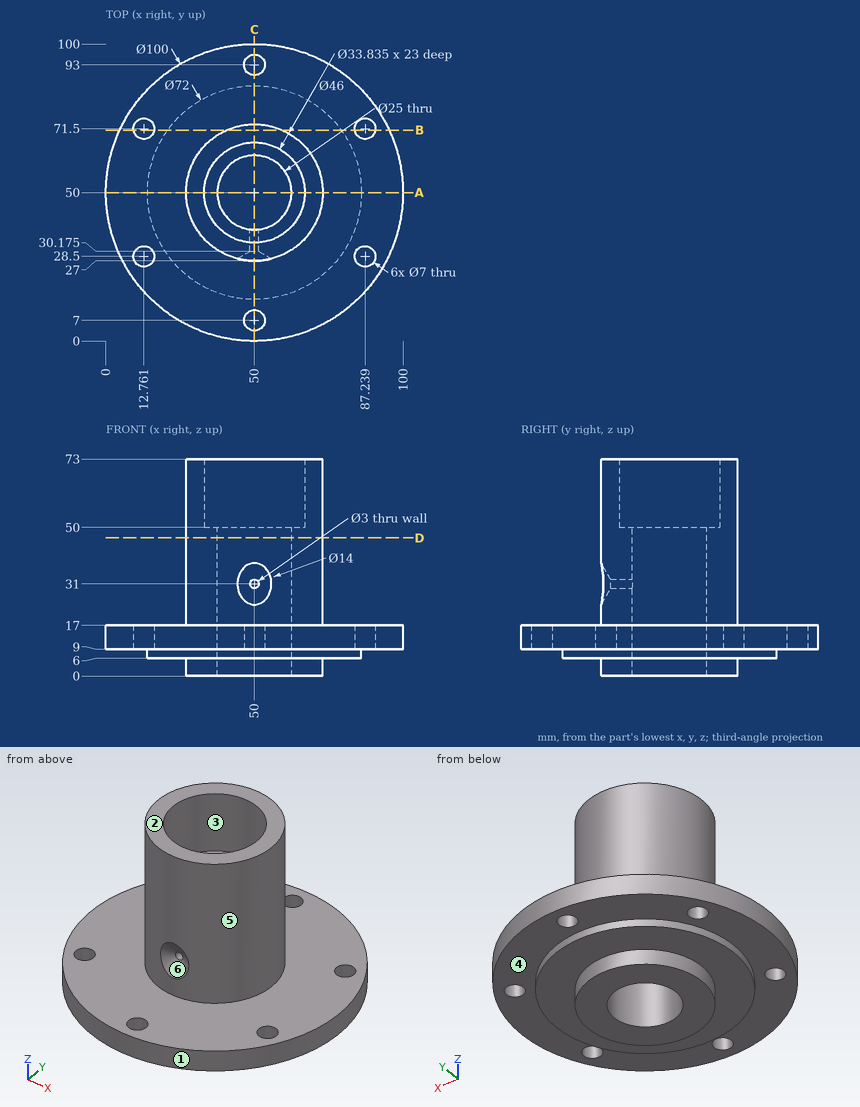
Answer from the drawing. Dimensions are ordinates in mm from the lowest x, y and z of the part. A direction names the side the tool comes from. Give positions to 0.01 mm unless a question says otherwise; leave off trailing zeros. Order: outer loops, then holes, each group sorted by start corner. A loop starts at its lowest first (then second) coordinate and runs counter-clockwise, first axis right, second up.
(1) Find section D-D (z = 46.5). Give the vertices of the cut face in (x, y).
(2) Find section C-C (x = 50). Give the number of separate pieces and of enclosed holes in the cut face, plus the area to 3 significant figures.
(3) Find section B-B (y = 71). Give the vertices of the cut face in (x, z) (1 decimal), plus the area to 3 significant figures.
(4) For a pull along X with two mould halves and no side action, classify the marked faces 1, 2 and 3 as released by +X, released by -X, zero draft, split by the parting line, or undercut.
(5) Given pin 1 (5 mm diameter, centred on x = 64, z = 33, fed in from -Y); pin 2 (9 mm diameter, centred on x = 87.24, y = 28.5, fed in from +Z); pin 3 (5 mm diameter, centred on y = 60.5, z = 43.5, fed in from -X); pin 4 (21.5 mm diameter, centred on x = 43.5, y = 45.5, fed in from -Z), each flat-ended and moving along its own axis, determine where each tip first touches the part or whether it passes through.
(6) For the marked faces 4, 5 and 6, determine the directions among +Z, -Z, +X, -X, +Y, -Y from which every point of the face is accessible in a straight line to the end or side of a thin tool.
(7) Find section A-A (y = 50). Give the vertices of the cut face in (x, z).
(8) Straight lines are drawn through the part: L1, parallel to X at y = 28, z = 12 (1 decimal); L2, parallel to X at y = 71.5, z = 12; L3, parallel to X at y = 50, z = 26.5. For each, find the intervals that lie inside material, in ascending order.
Result sheet:
1. outline: circle Ø46 at (50, 50); hole circle Ø25 at (50, 50)
2. separate pieces: 5
2. enclosed holes: 0
2. area: 1,680 mm2
3. outline: (4.6, 9) - (9.3, 9) - (9.3, 17) - (4.6, 17) - close; (16.2, 9) - (20.8, 9) - (20.8, 6) - (40.6, 6) - (40.6, 0) - (59.4, 0) - (59.4, 6) - (79.2, 6) - (79.2, 9) - (83.8, 9) - (83.8, 17) - (59.4, 17) - (59.4, 73) - (40.6, 73) - (40.6, 17) - (16.2, 17) - close; (90.7, 9) - (95.4, 9) - (95.4, 17) - (90.7, 17) - close
3. area: 1,950 mm2
4. face 1: split by the parting line
4. face 2: zero draft
4. face 3: undercut
5. pin 1: stops at y = 30.08
5. pin 2: stops at z = 17
5. pin 3: stops at x = 28.44
5. pin 4: stops at z = 0
6. face 4: -Z
6. face 5: +Z
6. face 6: -Y
7. outline: (0, 9) - (14, 9) - (14, 6) - (27, 6) - (27, 0) - (37.5, 0) - (37.5, 50) - (33.08, 50) - (33.08, 73) - (27, 73) - (27, 17) - (0, 17) - close; (62.5, 0) - (73, 0) - (73, 6) - (86, 6) - (86, 9) - (100, 9) - (100, 17) - (73, 17) - (73, 73) - (66.92, 73) - (66.92, 50) - (62.5, 50) - close
8. L1: x = 5.1 to 9.3, 16.2 to 83.8, 90.7 to 94.9
8. L2: x = 4.86 to 9.26, 16.26 to 83.74, 90.74 to 95.14
8. L3: x = 27 to 37.5, 62.5 to 73
